```python
from build123d import *

# Parameters (mm, degrees)
SKETCH1_R                = 21.082
SKETCH1_R_2              = 17.526
BOSS_EXTRUDE1_DEPTH      = 196.85
BOSS_EXTRUDE1_DEPTH_BACK = 196.85
SKETCH2_R                = 2.38125
CUT_EXTRUDE1_DEPTH       = 22.082
CUT_EXTRUDE1_DEPTH_BACK  = 22.082
SKETCH3_R                = 3.175
CUT_EXTRUDE2_DEPTH       = 22.0820001


with BuildPart() as part:
    # Sketch1 → Boss-Extrude1 (new body, two sides)
    with BuildSketch(Plane(origin=(0, 0, 0), x_dir=(0, 0, -1), z_dir=(1, 0, 0))) as boss_extrude1_sk:
        Circle(SKETCH1_R)
        Circle(SKETCH1_R_2, mode=Mode.SUBTRACT)
    extrude(amount=BOSS_EXTRUDE1_DEPTH)
    extrude(boss_extrude1_sk.sketch, amount=-BOSS_EXTRUDE1_DEPTH_BACK)

    # Sketch2 → Cut-Extrude1 (cut, two sides)
    with BuildSketch(Plane.XY) as cut_extrude1_sk:
        with Locations((-144.4625, 0)):
            Circle(SKETCH2_R)
        with Locations((-182.5625, 0)):
            Circle(SKETCH2_R)
    extrude(amount=CUT_EXTRUDE1_DEPTH, mode=Mode.SUBTRACT)
    extrude(cut_extrude1_sk.sketch, amount=-CUT_EXTRUDE1_DEPTH_BACK, mode=Mode.SUBTRACT)

    # Sketch3 → Cut-Extrude2 (cut, through all)
    with BuildSketch(Plane.XY):
        with Locations((165.1, 0)):
            Circle(SKETCH3_R)
        with Locations((114.3, 0)):
            Circle(SKETCH3_R)
    extrude(amount=CUT_EXTRUDE2_DEPTH, mode=Mode.SUBTRACT)


solid = part.part
```
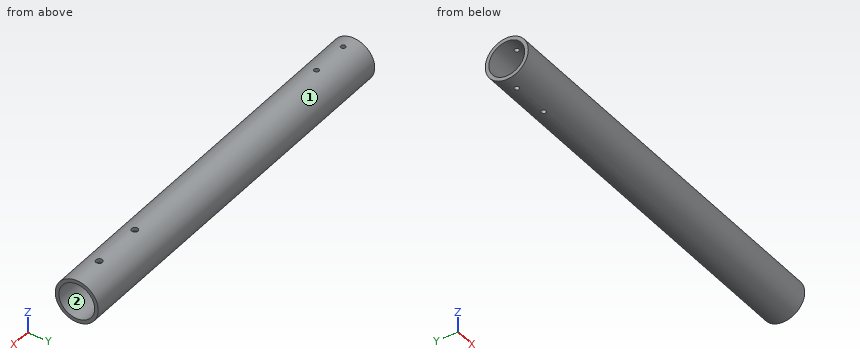
Input: part model. Units: mm. Frame: model coordinates. Face numbers are marked on the shaded views. Round coordinates to 2 decimals unless told otherwise and drop trailing zeros. Loops run counter-clockwise (first coordinate to the right, second up) from the corner with the lowest first, then second, coordinate; pieces in that order, holes last.
1) Material intervals for line 1 (X direction, y = 0, z = -18); line 2 (Z direction, x = -83, y = 0); line 3 (X direction, y = 1, z = 18.5), sorted ascending.
Ans:
line 1: x = -196.85 to -184.94, -180.18 to -146.84, -142.08 to 196.85
line 2: z = -21.08 to -17.53, 17.53 to 21.08
line 3: x = -196.85 to -184.72, -180.4 to -146.62, -142.3 to 111.29, 117.31 to 162.09, 168.11 to 196.85
2) Pull-direction query (Y, two-part tool) for the marked faces 1 and 2; classes: released by +Y, released by -Y, zero draft, split by the parting line, or undercut.
Ans:
face 1: split by the parting line
face 2: undercut
3) Pin query (flat end, axial travel): pin 1 (1 mm diameter, centred on y = -15.5, z = 16.5, fed in from -X); pin 2 (1.5 mm diameter, centred on x = 89, y = -16.5, fed in from +Z); pin 3 (4 mm diameter, centred on y = -4, z = 15.5, fed in from -X); pin 4 (4 mm diameter, centred on x = 103, y = 4, fed in from +Z). Return the tip coordinate at first contact, or that it passes through.
Ans:
pin 1: passes through
pin 2: stops at z = 14.01
pin 3: stops at x = -196.85
pin 4: stops at z = 20.99
4) Section query B-B on x = 80.5. Return the cut outline in (y, z), plus the area to 3 significant figures.
Ans:
outline: circle Ø42.16 at (0, 0); hole circle Ø35.05 at (0, 0)
area: 431 mm2
5) Section query A-A on z = 0. Return the cut outline in (x, y), plus the area to 3 significant figures.
Ans:
outline: (-196.85, -21.08) - (196.85, -21.08) - (196.85, -17.53) - (-196.85, -17.53) - close; (-196.85, 17.53) - (196.85, 17.53) - (196.85, 21.08) - (-196.85, 21.08) - close
area: 2,800 mm2
